Design review of the part built by this model. Coordinates are the model's own, in mm. Coordinates: 2 decimals unless noted, no trailing zeros. Write each loop counter-clockwise with the first axis right and the second up, starting at its lowest first coordinate (ties: lowest second). Pieces come first, ordered by that corner, then holes.
Q1. For L1, parallel to X at y = 1.15, z = -20; L2, parallel to Z at x = 14, y = 2.75; L3, parallel to X at y = 1.2, z = -26, list the stretches that pass through material, from the lowest coordinate up.
Q2. Take a section at B-B, the plane z = -14. Write out the cut boundary in (x, y), plus the area to 3 significant figures.
Q3. The part is to be moulded in two halves that separate along X. For faces 1 (the flat face through (0, 2, -20)), 2 (the flat face through (20, 2, 0)), 3 (the cylindrical face through (14, 3, -19)), say which applies: released by +X, released by -X, zero draft, split by the parting line, or undercut.
Q4. Take a section at C-C, the plane x = 26. Write out the cut boundary in (y, z), plus the area to 3 significant figures.
Q5. Take a section at D-D, the plane y = 3.85. Write out the cut boundary in (x, z).
Q6. Take a section at A-A, the plane x = 20. Write out the cut boundary in (y, z), plus the area to 3 significant figures.
from build123d import *

# Parameters (mm, degrees)
SKETCH1_W               = 40
SKETCH1_H               = 40
BOSS_EXTRUDE1_DEPTH     = 5
SKETCH8_R               = 3
SKETCH8_R_2             = 1
CUT_EXTRUDE4_DEPTH      = 15
CUT_EXTRUDE4_DEPTH_BACK = 15


with BuildPart() as part:
    # Sketch1 → Boss-Extrude1 (new body)
    with BuildSketch(Plane(origin=(0, 0, 0), x_dir=(1, 0, 0), z_dir=(0, 1, 0))):
        with Locations((20, 20)):
            Rectangle(SKETCH1_W, SKETCH1_H)
    extrude(amount=BOSS_EXTRUDE1_DEPTH)

    # Sketch8 → Cut-Extrude4 (cut, two sides)
    with BuildSketch(Plane(origin=(0, 5, 0), x_dir=(1, 0, 0), z_dir=(0, 1, 0))) as cut_extrude4_sk:
        with Locations((20, 20)):
            Circle(SKETCH8_R)
        with Locations((20, 14)):
            Circle(SKETCH8_R_2)
        with Locations((26, 20)):
            Circle(SKETCH8_R_2)
        with Locations((14, 20)):
            Circle(SKETCH8_R_2)
        with Locations((20, 26)):
            Circle(SKETCH8_R_2)
    extrude(amount=CUT_EXTRUDE4_DEPTH, mode=Mode.SUBTRACT)
    extrude(cut_extrude4_sk.sketch, amount=-CUT_EXTRUDE4_DEPTH_BACK, mode=Mode.SUBTRACT)


solid = part.part
Responses:
1. L1: x = 0 to 13, 15 to 17, 23 to 25, 27 to 40
1. L2: z = -40 to -21, -19 to 0
1. L3: x = 0 to 19, 21 to 40
2. outline: (0, 0) - (19, 0) - (19, 5) - (0, 5) - close; (21, 0) - (40, 0) - (40, 5) - (21, 5) - close
2. area: 190 mm2
3. face 1: released by -X
3. face 2: zero draft
3. face 3: undercut
4. outline: (0, -40) - (5, -40) - (5, -21) - (0, -21) - close; (0, -19) - (5, -19) - (5, 0) - (0, 0) - close
4. area: 190 mm2
5. outline: (0, -40) - (40, -40) - (40, 0) - (0, 0) - close; hole circle Ø2 at (14, -20); hole circle Ø6 at (20, -20); hole circle Ø2 at (20, -26); hole circle Ø2 at (20, -14); hole circle Ø2 at (26, -20)
6. outline: (0, -40) - (5, -40) - (5, -27) - (0, -27) - close; (0, -25) - (5, -25) - (5, -23) - (0, -23) - close; (0, -17) - (5, -17) - (5, -15) - (0, -15) - close; (0, -13) - (5, -13) - (5, 0) - (0, 0) - close
6. area: 150 mm2
